CAD build for the part. Positions are in the model's coordinates, mm. Face numbers are marked on the shaded views. A direction names the side the tool comes from. Give positions to 0.01 mm unless a question says otherwise; leave off trailing zeros. Loops run counter-clockwise (first coordinate to the right, second up) from the corner with the lowest first, then second, coordinate; pieces in that order, holes last. Notation, with made-up numbers: M 3,49.25 L 31,49.25 A23 ccw 31,80.25 Z; hole C 25.5,79.5 d10. An arc over 180 degrees is marked long. Answer as CSV lines item,"result".
```python
from build123d import *

# Parameters (mm, degrees)
BASE_FLANGE1_DEPTH = 50.8
SKETCH7_R          = 4.826
CUT_EXTRUDE1_DEPTH = 2.54
SKETCH8_R          = 4.826
CUT_EXTRUDE2_DEPTH = 2.54


# Sheet-metal steps are written as plain solids
with BuildPart() as part:
    # Sketch2 → Base-Flange1 (new body)
    with BuildSketch(Plane.XY):
        with BuildLine():
            Line((-72.359580073, 0), (15.803819927, 0))
            ThreePointArc((15.803819927, 0), (25.304930904, -3.935489024), (29.240419927, -13.4366))
            Line((29.240419927, -13.4366), (29.240419927, -50.8))
            Line((29.240419927, -50.8), (28.503819927, -50.8))
            Line((28.503819927, -50.8), (28.503819927, -13.4366))
            ThreePointArc((28.503819927, -13.4366), (24.784076049, -4.456343879), (15.803819927, -0.7366))
            Line((15.803819927, -0.7366), (-72.359580073, -0.7366))
            Line((-72.359580073, -0.7366), (-72.359580073, 0))
        make_face()
    extrude(amount=BASE_FLANGE1_DEPTH)

    # Sketch7 → Cut-Extrude1 (cut)
    with BuildSketch(Plane(origin=(29.240419927, 0, 0), x_dir=(0, 0, -1), z_dir=(1, 0, 0))):
        with Locations(Location((-12.894872644, -32.1183, 0), (0, 0, 90))):
            Circle(SKETCH7_R)
        with Locations(Location((-38.294872644, -32.1183, 0), (0, 0, 90))):
            Circle(SKETCH7_R)
    extrude(amount=-CUT_EXTRUDE1_DEPTH, mode=Mode.SUBTRACT)

    # Sketch8 → Cut-Extrude2 (cut)
    with BuildSketch(Plane(origin=(0, 0, 0), x_dir=(1, 0, 0), z_dir=(0, 1, 0))):
        with Locations(Location((-28.277880073, -38.1, 0), (0, 0, 270))):
            Circle(SKETCH8_R)
        with Locations(Location((-28.277880073, -12.7, 0), (0, 0, 270))):
            Circle(SKETCH8_R)
    extrude(amount=-CUT_EXTRUDE2_DEPTH, mode=Mode.SUBTRACT)


solid = part.part
```
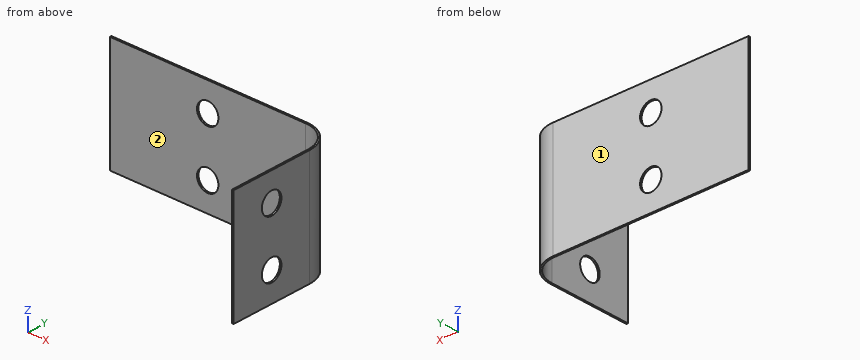
Q1. Cut at D-D (y = -16). Write the cut outline in (x, z).
Solution:
outline,"M 28.5,0 L 29.24,0 L 29.24,50.8 L 28.5,50.8 Z"
Q2. Cut at A-A (z = 10). Write the cut outline in (x, y), and give its area (3 significant figures).
Solution:
outline,"M -72.36,-0.74 L -32.28,-0.74 L -32.28,0 L -72.36,0 Z; M -24.28,-0.74 L 15.8,-0.74 A12.7 cw 28.5,-13.44 L 28.5,-28.26 L 29.24,-28.26 L 29.24,-13.44 A13.44 ccw 15.8,0 L -24.28,0 Z; M 28.5,-50.8 L 29.24,-50.8 L 29.24,-35.98 L 28.5,-35.98 Z"
area,"96.0 mm²"
Q3. Pin check, flat tips, straight feed: P1, Ø15.5, axis at x = -28.28, z = 12.7, coming from the +Y side; P2, Ø8, axis at x = 7, z = 12.5, coming from the -Y side; P3, Ø12, axis at y = -45, z = 33, coming from the -X side. Stop position of each tip, or through.
Solution:
P1,"stops at y = 0"
P2,"stops at y = -0.74"
P3,"stops at x = 28.5"
Q4. Which spindle directions (+Z, -Z, +X, -X, +Y, -Y) get a long thin tool onto all of the face, cutting with end or side? Do the marked faces 1 and 2. Say none if no direction does.
Solution:
face 1,"+Z, -Z, +X, -X, +Y"
face 2,"+Z, -Z, -X, -Y"
Q5. Wall check: line 1 (X direction, y = -17, z = 33); line 2 (Y direction, x = -34.5, z = 40.5); line 3 (X direction, y = -8.5, z = 36). Give the ranges that are in metal, low to high. Write a range as [from, to].
Solution:
line 1,"x = [28.5, 29.24]"
line 2,"y = [-0.74, 0]"
line 3,"x = [27.51, 28.3]"
Q6. Cut at C-C (x = -25). Write the cut outline in (y, z).
Solution:
outline,"M -0.74,0 L 0,0 L 0,9.16 L -0.74,9.16 Z; M -0.74,16.24 L 0,16.24 L 0,34.56 L -0.74,34.56 Z; M -0.74,41.64 L 0,41.64 L 0,50.8 L -0.74,50.8 Z"
Q7. Cut at B-B (z = 32). Write the cut outline in (x, y).
Solution:
outline,"M -72.36,-0.74 L 15.8,-0.74 A12.7 cw 28.5,-13.44 L 28.5,-50.8 L 29.24,-50.8 L 29.24,-13.44 A13.44 ccw 15.8,0 L -72.36,0 Z"
